Study the drawing (mm; zero at the part's minimum x, y, z) and answer. A direction names the side the tool comes from. Coordinates: 2 decimals unless noted, no trailing zeros. Order: outer loops, then holes, each group sorted by start corner. A loop starts at its lowest first (then second) coordinate and runs counter-clockwise, first axis right, second up.
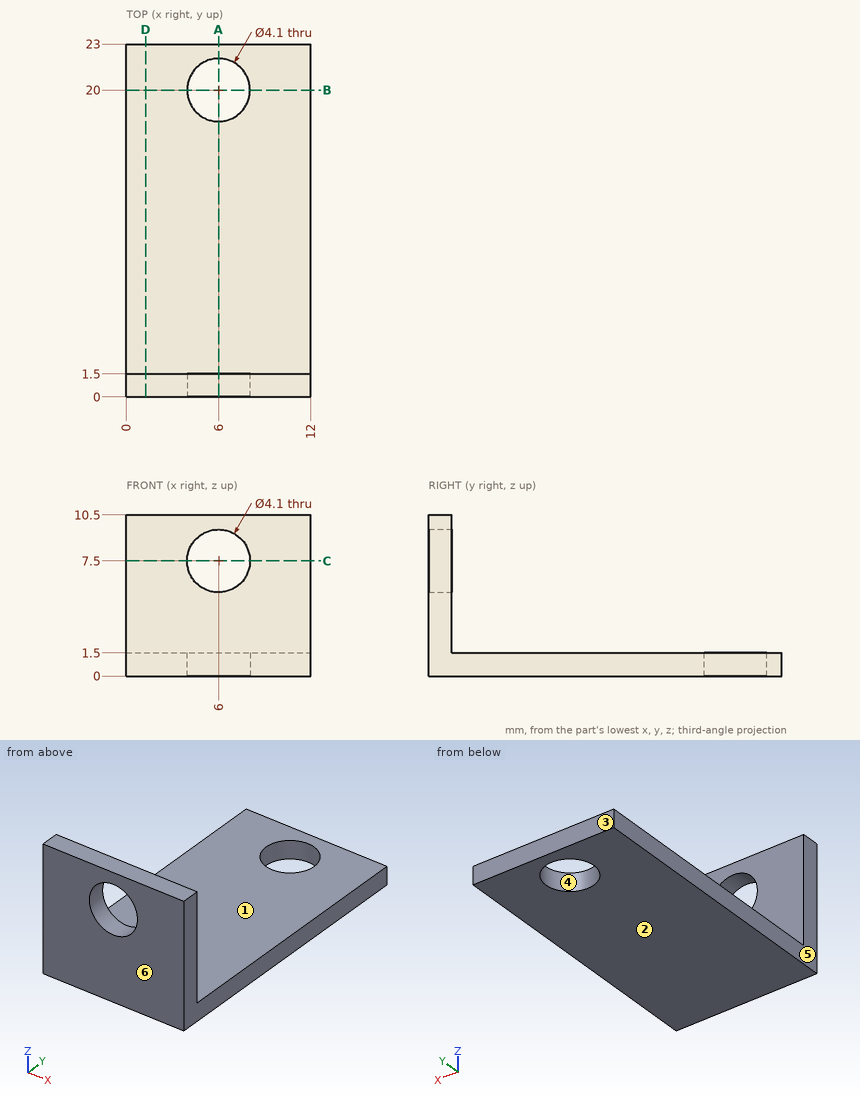
1) Flat-ended cylindrical pins translate along their axes: pin 1 Ø1.5 at (x, z) = (7.5, 3) entering from +Y; pin 2 Ø3.5 at (x, z) = (6, 7.5) entering from +Y; pin 3 Ø6.5 at (x, y) = (6, 20) entering from +Z. Find the tip coordinate at first contact, or state that the pin passes through.
A:
pin 1: stops at y = 1.5
pin 2: passes through
pin 3: stops at z = 1.5
2) Determine the mould class of the marked faces 3, 4, 5 and 6 for opening direction Y: pulls with the +Y half, pulls with the -Y half, needs draft (parallel to the pull), parting line crosses it, or undercut.
A:
face 3: pulls with the +Y half
face 4: undercut
face 5: needs draft
face 6: pulls with the -Y half
3) A cutting plane is placed at B-B, the plane y = 20. Determine the outline of the cut face in (x, z).
A:
outline: (0, 0) - (3.95, 0) - (3.95, 1.5) - (0, 1.5) - close; (8.05, 0) - (12, 0) - (12, 1.5) - (8.05, 1.5) - close
4) A cutting plane is placed at A-A, the plane x = 6. Determine the outline of the cut face in (y, z).
A:
outline: (0, 0) - (17.95, 0) - (17.95, 1.5) - (1.5, 1.5) - (1.5, 5.45) - (0, 5.45) - close; (0, 9.55) - (1.5, 9.55) - (1.5, 10.5) - (0, 10.5) - close; (22.05, 0) - (23, 0) - (23, 1.5) - (22.05, 1.5) - close
5) Which of the six approach directions +Z, -Z, +X, -X, +Y, -Y give full straight-line access (tool end or side, diameter ignored) to the marked faces 1 and 2?
A:
face 1: +Z, +X, -X, +Y
face 2: -Z, +X, -X, +Y, -Y
6) Straight lines are drawn through the part: line 1 (Y direction, x = 6, z = 1.05); line 2 (Z direction, x = 6, y = 0.6); line 3 (Y direction, x = 10.5, z = 8.75). For each, find the intervals that lie inside material, in ascending order.
A:
line 1: y = 0 to 17.95, 22.05 to 23
line 2: z = 0 to 5.45, 9.55 to 10.5
line 3: y = 0 to 1.5
7) A cutting plane is placed at D-D, the plane x = 1.25. Determine the outline of the cut face in (y, z).
A:
outline: (0, 0) - (23, 0) - (23, 1.5) - (1.5, 1.5) - (1.5, 10.5) - (0, 10.5) - close
